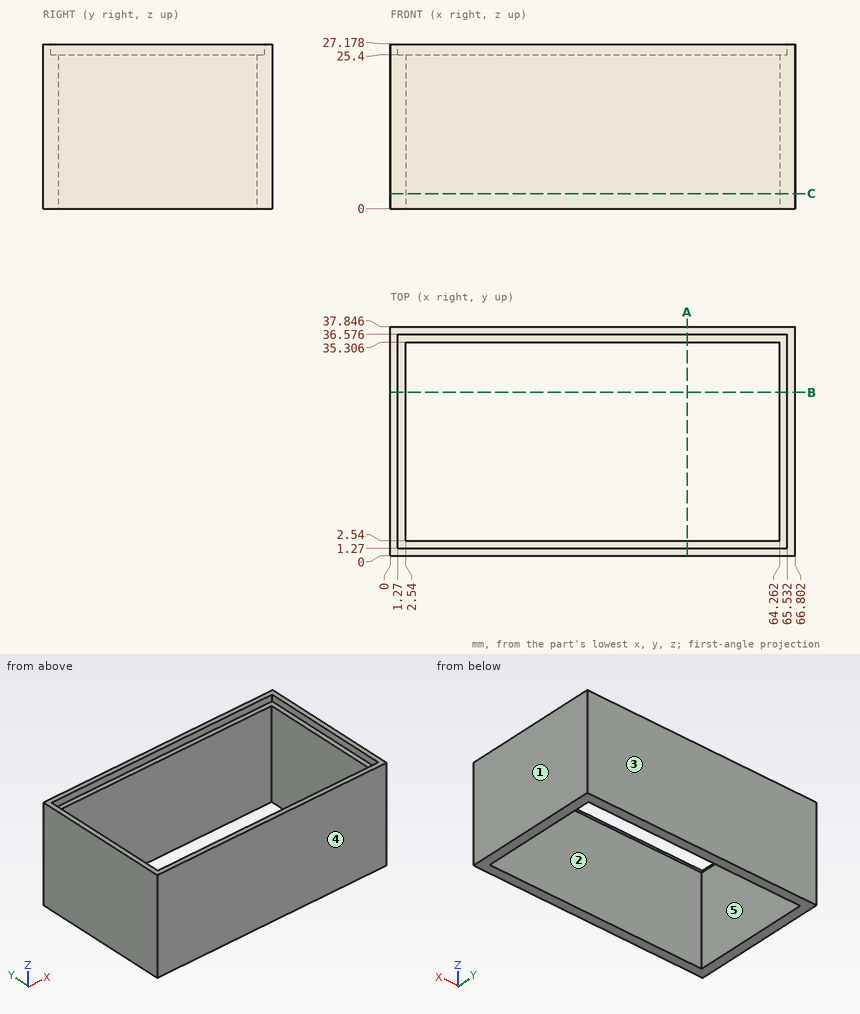
Input: dimensioned drawing with shaded views. Units: mm. Origin: part minimum x, y, z. A direction names the side the tool comes from. Coordinates: 2 decimals unless noted, no trailing zeros. Order: outer loops, then holes, each group sorted by start corner. A loop starts at its lowest first (then second) coordinate and runs counter-clockwise, first axis right, second up.
(1) Section query C-C (z = 2.5). Return the cut outline in (x, y), plus the area to 3 significant figures.
(2) Section query A-A (x = 49). Return the cut outline in (y, z), plus the area to 3 significant figures.
(3) Section query B-B (y = 27). Return the cut outline in (x, z).
(4) Access query for the marked faces 4 and 5. Directions: +Z, -Z, +X, -X, +Y, -Y. A direction counts if a zero-diameter tool reaches every point of the face in a straight line with its end or side. Return the directions, or none.
(5) Draft query along X for the marked faces 1, 2 and 3. Return one class per face: pulls with the +X half, pulls with the -X half, needs draft (parallel to the pull), parting line crosses it, or undercut.
(6) Material intervals for probe 1 along X at (y, z) = (17, 16.5); probe 2 along Y at (x, z) = (22, 9.5), sorted ascending.
Solution:
1. outline: (0, 0) - (66.8, 0) - (66.8, 37.85) - (0, 37.85) - close; hole (2.54, 2.54) - (64.26, 2.54) - (64.26, 35.31) - (2.54, 35.31) - close
1. area: 506 mm2
2. outline: (0, 0) - (2.54, 0) - (2.54, 25.4) - (1.27, 25.4) - (1.27, 27.18) - (0, 27.18) - close; (35.31, 0) - (37.85, 0) - (37.85, 27.18) - (36.58, 27.18) - (36.58, 25.4) - (35.31, 25.4) - close
2. area: 134 mm2
3. outline: (0, 0) - (2.54, 0) - (2.54, 25.4) - (1.27, 25.4) - (1.27, 27.18) - (0, 27.18) - close; (64.26, 0) - (66.8, 0) - (66.8, 27.18) - (65.53, 27.18) - (65.53, 25.4) - (64.26, 25.4) - close
4. face 4: +Z, -Z, +X, -X, -Y
4. face 5: +Z, -Z
5. face 1: pulls with the +X half
5. face 2: undercut
5. face 3: needs draft
6. probe 1: x = 0 to 2.54, 64.26 to 66.8
6. probe 2: y = 0 to 2.54, 35.31 to 37.85
